```python
from build123d import *

# Parameters (mm, degrees)
BOSS_EXTRU_1_DEPTH      = 10
ENL_V_MAT_EXTRU_1_DEPTH = 20
ENL_V_MAT_EXTRU_2_DEPTH = 20
ESQUISSE5_R             = 1.6
ENL_V_MAT_EXTRU_3_DEPTH = 20
ESQUISSE6_R             = 1.6
ENL_V_MAT_EXTRU_4_DEPTH = 20
CHANFREIN1_SIZE         = 2
ENL_V_MAT_EXTRU_5_DEPTH = 2
ENL_V_MAT_EXTRU_6_DEPTH = 2
ESQUISSE9_R             = 1.6
ENL_V_MAT_EXTRU_7_DEPTH = 10


with BuildPart() as part:
    # Esquisse1 → Boss.-Extru.1 (new body)
    with BuildSketch(Plane.XY):
        with BuildLine():
            Line((-20, 102.058806577), (0, 102.058806577))
            Line((0, 102.058806577), (0, 91.847700026))
            Line((0, 91.847700026), (-20, 91.847700026))
            ThreePointArc((-20, 91.847700026), (-66.468037432, 66.468037432), (-91.847700026, 20))
            Line((-91.847700026, 20), (-91.847700026, 0))
            Line((-91.847700026, 0), (-102.058806577, 0))
            Line((-102.058806577, 0), (-102.058806577, 20))
            ThreePointArc((-102.058806577, 20), (-73.539105243, 73.539105243), (-20, 102.058806577))
        make_face()
    extrude(amount=BOSS_EXTRU_1_DEPTH)

    # Esquisse2 → Enlèv. mat.-Extru.1 (cut)
    with BuildSketch(Plane.XZ):
        Polygon((-98.847700026, 10), (-91.847700026, 10), (-91.847700026, 0), (-98.847700026, 0), (-95.847700026, 2.5), (-95.847700026, 7.5), align=None)
    extrude(amount=-ENL_V_MAT_EXTRU_1_DEPTH, mode=Mode.SUBTRACT)

    # Esquisse4 → Enlèv. mat.-Extru.2 (cut)
    with BuildSketch(Plane(origin=(0, 0, 0), x_dir=(0, 0, -1), z_dir=(1, 0, 0))):
        Polygon((0, 98.847700026), (0, 91.847700026), (-10, 91.847700026), (-10, 98.847700026), (-7.5, 95.847700026), (-2.5, 95.847700026), align=None)
    extrude(amount=-ENL_V_MAT_EXTRU_2_DEPTH, mode=Mode.SUBTRACT)

    # Esquisse5 → Enlèv. mat.-Extru.3 (cut)
    with BuildSketch(Plane(origin=(-95.847700026, 0, 0), x_dir=(0, 0, -1), z_dir=(1, 0, 0))):
        with Locations(Location((-5, 5, 0), (0, 0, 90))):
            Circle(ESQUISSE5_R)
        with Locations(Location((-5, 15, 0), (0, 0, 90))):
            Circle(ESQUISSE5_R)
    extrude(amount=-ENL_V_MAT_EXTRU_3_DEPTH, mode=Mode.SUBTRACT)

    # Esquisse6 → Enlèv. mat.-Extru.4 (cut)
    with BuildSketch(Plane.XZ.offset(-95.847700026)):
        with Locations(Location((-5, 5.05896145, 0), (0, 0, 270))):
            Circle(ESQUISSE6_R)
        with Locations(Location((-15, 5.05896145, 0), (0, 0, 270))):
            Circle(ESQUISSE6_R)
    extrude(amount=-ENL_V_MAT_EXTRU_4_DEPTH, mode=Mode.SUBTRACT)

    # Chanfrein1
    chanfrein1_edges = [part.edges().sort_by_distance(p)[0] for p in [
        (-97.347700026, 0, 8.75),
        (-95.847700026, 0, 5),
        (-97.347700026, 0, 1.25),
        (0, 97.347700026, 1.25),
        (0, 95.847700026, 5),
        (0, 97.347700026, 8.75),
    ]]
    chamfer(chanfrein1_edges, length=CHANFREIN1_SIZE)

    # Esquisse7 → Enlèv. mat.-Extru.5 (cut)
    with BuildSketch(Plane.ZY.offset(102.058806577)):
        Polygon((2.2, 6.616580754), (2.2, 3.383419246), (5, 1.766838493), (7.8, 3.383419246), (7.8, 6.616580754), (5, 8.233161507), align=None)
        Polygon((7.8, 16.616580754), (5, 18.233161507), (2.2, 16.616580754), (2.2, 13.383419246), (5, 11.766838493), (7.8, 13.383419246), align=None)
    extrude(amount=-ENL_V_MAT_EXTRU_5_DEPTH, mode=Mode.SUBTRACT)

    # Esquisse8 → Enlèv. mat.-Extru.6 (cut)
    with BuildSketch(Plane(origin=(0, 102.058806577, 0), x_dir=(1, 0, 0), z_dir=(0, 1, 0))):
        Polygon((-3.383419246, -2.25896145), (-6.616580754, -2.25896145), (-8.233161507, -5.05896145), (-6.616580754, -7.85896145), (-3.383419246, -7.85896145), (-1.766838493, -5.05896145), align=None)
        Polygon((-13.383419246, -2.25896145), (-16.616580754, -2.25896145), (-18.233161507, -5.05896145), (-16.616580754, -7.85896145), (-13.383419246, -7.85896145), (-11.766838493, -5.05896145), align=None)
    extrude(amount=-ENL_V_MAT_EXTRU_6_DEPTH, mode=Mode.SUBTRACT)

    # Esquisse9 → Enlèv. mat.-Extru.7 (cut)
    with BuildSketch(Plane(origin=(0, 0, 0), x_dir=(-1, 0, 0), z_dir=(0, 0, -1))):
        with Locations((94.345111161, 30)):
            Circle(ESQUISSE9_R)
        with Locations((90.837371891, 39.364601711)):
            Circle(ESQUISSE9_R)
        with Locations((30, 94.345111161)):
            Circle(ESQUISSE9_R)
        with Locations((39.364601711, 90.837371891)):
            Circle(ESQUISSE9_R)
    extrude(amount=-ENL_V_MAT_EXTRU_7_DEPTH, mode=Mode.SUBTRACT)


solid = part.part
```
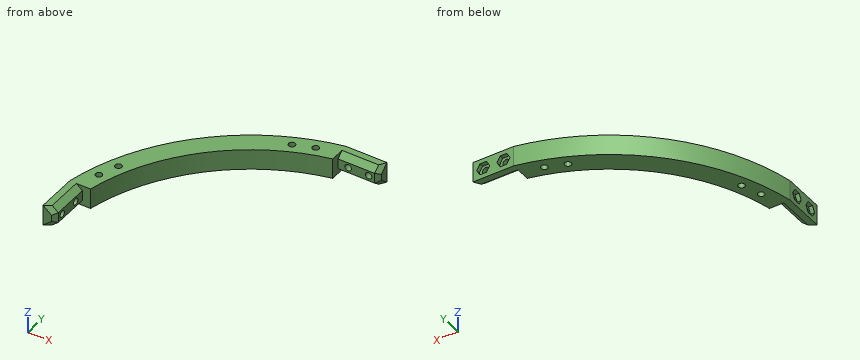
Input: part model. Units: mm. Frame: model coordinates. Coordinates: 2 decimals unless noted, no trailing zeros. Order: outer loops, then holes, each group sorted by start corner. A loop starts at its lowest first (then second) coordinate and runs counter-clockwise, first axis right, second up. Notation, with made-up numbers: (38.25, 5) - (59.25, 5) arc R19 cw to (59.25, 34) - close; hole circle Ø10 at (-8, -27.5). An arc over 180 degrees is marked (long way). Put each result on its own line as item: value.
1. Cut plane D-D on y = 46.5. Return the cut outline in (x, z), then the cut area to 3 significant figures.
Report:
outline: (-93.03, 0) - (-81.69, 0) - (-81.69, 10) - (-93.03, 10) - close
area: 113 mm2
2. Cut plane A-A on y = 15. Return the cut outline in (x, z), then the cut area to 3 significant figures.
Report:
outline: (-102.06, 0) - (-98.85, 0) - (-95.85, 2.5) - (-95.85, 3.4) - (-100.06, 3.4) - (-100.06, 2.2) - (-102.06, 2.2) - close; (-102.06, 7.8) - (-100.06, 7.8) - (-100.06, 6.6) - (-95.85, 6.6) - (-95.85, 7.5) - (-98.85, 10) - (-102.06, 10) - close
area: 29.9 mm2
3. Cut plane B-B on x = -5. Return the cut outline in (y, z).
Report:
outline: (95.85, 2.5) - (98.85, 0) - (102.06, 0) - (102.06, 2.26) - (100.06, 2.26) - (100.06, 3.46) - (95.85, 3.46) - close; (95.85, 6.66) - (100.06, 6.66) - (100.06, 7.86) - (102.06, 7.86) - (102.06, 10) - (98.85, 10) - (95.85, 7.5) - close
4. Cut plane C-C on x = -30. Return the cut outline in (y, z).
Report:
outline: (89.08, 0) - (92.75, 0) - (92.75, 10) - (89.08, 10) - close; (95.95, 0) - (99.58, 0) - (99.58, 10) - (95.95, 10) - close
5. Line query: line 1 along Z through (x, y) = (-99.05, 5); line 2 along Y through (x, z) = (-30, 2.5); line 3 along Y through (x, z) = (-85, 2.75). Output: solid intervals per line, ascending.
Report:
line 1: z = 0 to 3.4, 6.6 to 10
line 2: y = 89.08 to 92.75, 95.95 to 99.58
line 3: y = 40.14 to 59.92
6. Contact query for flat-ended pins moving along their axis: pin 1 Ø4 at (y, z) = (80.5, 4.5) entering from +X; pin 2 Ø2 at (y, z) = (65, 5) entering from +X; pin 3 Ø4 at (y, z) = (63.5, 7.5) entering from +X; pin 4 Ø3.5 at (x, y) = (-94.35, 30) entering from -Z. Output: stop coordinate, or through.
Report:
pin 1: stops at x = -45.05
pin 2: stops at x = -66.93
pin 3: stops at x = -67.42
pin 4: stops at z = 0
